from build123d import *

# Parameters (mm, degrees)
CHAMFER1_SIZE = 0.5


with BuildPart() as part:
    # Sketch2 → Revolve1 (revolve)
    with BuildSketch(Plane(origin=(0, 0, 0), x_dir=(0, 0, -1), z_dir=(1, 0, 0))):
        with BuildLine():
            Line((65.5, 0), (-5, 0))
            Line((-5, 0), (-5.7, 0))
            ThreePointArc((-5.7, 0), (-5.513084713, -0.716327439), (-5, -1.25))
            Line((-5, -1.25), (0, -1.25))
            Line((0, -1.25), (0, -2))
            Line((0, -2), (60.5, -2))
            Line((60.5, -2), (60.5, -1.25))
            Line((60.5, -1.25), (65.5, -1.25))
            ThreePointArc((65.5, -1.25), (66.013084713, -0.716327439), (66.2, 0))
            Line((66.2, 0), (65.5, 0))
        make_face()
    revolve(axis=Axis((0, 0, -65.5), (0, 0, 1)))

    # Chamfer1
    chamfer1_edges = [part.edges().sort_by_distance(p)[0] for p in [
        (0, 2, -60.5),
        (0, 2, 0),
    ]]
    chamfer(chamfer1_edges, length=CHAMFER1_SIZE)


solid = part.part
Verification items for the finished model (mm, model axes). A direction names the side the tool comes from. Give positions to 0.01 mm unless a question says otherwise; leave off trailing zeros. Loops run counter-clockwise (first coordinate to the right, second up) from the corner with the lowest first, then second, coordinate; pieces in that order, holes last.
1. Tool access check on faces 1 (the cylindrical face through (-2, 0, -31)), 2 (the cylindrical face through (-1.22, 0.27, -63.04)), 3 (the cylindrical face through (-1.22, 0.27, 2.46)). Record the directions out of +Z, -Z, +X, -X, +Y, -Y that give a thin tool (end or side, any length) a straight path to the whole face; none if there is none.
Derived:
face 1: +Z, -Z
face 2: -Z
face 3: +Z
2. Cross-section at A-A on y = 0. Record the cut outline in (x, z), and give its area (3 significant figures).
Derived:
outline: (-2, -60) - (-1.5, -60.5) - (-1.25, -60.5) - (-1.25, -65.5) arc R1.47 ccw to (1.25, -65.5) - (1.25, -60.5) - (1.5, -60.5) - (2, -60) - (2, -0.5) - (1.5, 0) - (1.25, 0) - (1.25, 5) arc R1.47 ccw to (-1.25, 5) - (-1.25, 0) - (-1.5, 0) - (-2, -0.5) - close
area: 269 mm2
3. Go/stop test with a flat-tipped pin: P1, Ø1, axis at x = -1.5, y = 0, coming from the +Z side. Record where the tip stops, or that it passes through.
Derived:
P1: stops at z = 5.31
4. Cross-section at C-C on z = -44.5. Record the cut outline in (x, y), and give its area (3 significant figures).
Derived:
outline: circle Ø4 at (0, 0)
area: 12.6 mm2
5. Material ranges on probe 1 along X at (y, z) = (1.55, -31.5); probe 2 along Y at (x, z) = (-0.1, -57); probe 3 along X at (y, z) = (0.1, -61), recorded low to high.
Derived:
probe 1: x = -1.26 to 1.26
probe 2: y = -2 to 2
probe 3: x = -1.25 to 1.25
